Verification items for the finished model (mm, model axes). A direction names the side the tool comes from. Coordinates: 2 decimals unless noted, no trailing zeros. Order: outer loops, then holes, each group sorted by start corner. A loop starts at its lowest first (then second) coordinate and runs counter-clockwise, first axis right, second up. Notation, with made-up numbers: (10.5, -39.75) -> (49.5, -39.75) arc R18 ccw to (49.5, -14.75) -> close; hole circle Ø9 at (86, 50). An arc over 180 degrees is marked (long way). Use CSV: the item, a comma, the result in double quotes. Start each with the question number.
1) Scan line: line 1 along X through (y, z) = (-5.75, 2.75). Record every from-to range of solid material in increasing order.
2) Sectioned sample at B-B on y = -4.75. Record the boundary of the cut face in (x, z), then the cut area to 3 significant figures.
3) Release check for a two-part mould opening along Y. For faces 4 (the flat face through (26, 0.1, 2)), 5 (the flat face through (0, 7.1, 1)), 6 (the flat face through (-26, 0.1, 2)), 7 (the flat face through (27.5, -1, 1)) record: released by +Y, released by -Y, zero draft, split by the parting line, or undercut.
4) Go/stop test with a flat-tipped pin: pin 1 (0.9 mm diameter, centred on y = 2.5, z = 1, fed in from +X). Record where the tip stops, or that it passes through.
5) Sectioned sample at A-A on z = 2. Record the boundary of the cut face in (x, y).
6) Tool access check on faces 1 (the flat face through (26, -6.9, 2)), 2 (the flat face through (-24.5, 2, 2)), 3 (the flat face through (0, -7.1, 1)). Record the directions out of +Z, -Z, +X, -X, +Y, -Y that give a thin tool (end or side, any length) a straight path to the whole face; none if there is none.
from build123d import *

# Parameters (mm, degrees)
SKETCH1_W           = 55
SKETCH1_H           = 14.2
BOSS_EXTRUDE1_DEPTH = 3
SKETCH3_W           = 3
SKETCH3_H           = 4
CUT_EXTRUDE1_DEPTH  = 10
SKETCH4_W           = 3
SKETCH4_H           = 4
CUT_EXTRUDE2_DEPTH  = 10


with BuildPart() as part:
    # Sketch1 → Boss-Extrude1 (new body)
    with BuildSketch(Plane.XY):
        Rectangle(SKETCH1_W, SKETCH1_H)
    extrude(amount=BOSS_EXTRUDE1_DEPTH)

    # Sketch3 → Cut-Extrude1 (cut)
    with BuildSketch(Plane.XY.offset(3)):
        with Locations((-26, 2.1)):
            Rectangle(SKETCH3_W, SKETCH3_H)
        with Locations((-26, -4.9)):
            Rectangle(SKETCH3_W, SKETCH3_H)
    extrude(amount=-CUT_EXTRUDE1_DEPTH, mode=Mode.SUBTRACT)

    # Sketch4 → Cut-Extrude2 (cut)
    with BuildSketch(Plane.XY.offset(3)):
        with Locations((26, 2.1)):
            Rectangle(SKETCH4_W, SKETCH4_H)
        with Locations((26, -4.9)):
            Rectangle(SKETCH4_W, SKETCH4_H)
    extrude(amount=-CUT_EXTRUDE2_DEPTH, mode=Mode.SUBTRACT)


solid = part.part
Answers follow:
1,line 1,"x = -24.5 to 24.5"
2,outline,"(-24.5, 0) -> (24.5, 0) -> (24.5, 3) -> (-24.5, 3) -> close"
2,area,"147 mm²"
3,face 4,"undercut"
3,face 5,"released by +Y"
3,face 6,"undercut"
3,face 7,"zero draft"
4,pin 1,"stops at x = 24.5"
5,outline,"(-27.5, -7.1) -> (27.5, -7.1) -> (27.5, -6.9) -> (24.5, -6.9) -> (24.5, -2.9) -> (27.5, -2.9) -> (27.5, 0.1) -> (24.5, 0.1) -> (24.5, 4.1) -> (27.5, 4.1) -> (27.5, 7.1) -> (-27.5, 7.1) -> (-27.5, 4.1) -> (-24.5, 4.1) -> (-24.5, 0.1) -> (-27.5, 0.1) -> (-27.5, -2.9) -> (-24.5, -2.9) -> (-24.5, -6.9) -> (-27.5, -6.9) -> close"
6,face 1,"+Z, -Z, +X"
6,face 2,"+Z, -Z, -X"
6,face 3,"+Z, -Z, +X, -X, -Y"
